Autodesk Inventor part; units mm, degrees
ref_plane "YZ Plane" through (0, 0, 0) normal (1, 0, 0) x (0, 1, 0)
ref_plane "XZ Plane" through (0, 0, 0) normal (0, 1, 0) x (-1, 0, 0)
ref_plane "XY Plane" through (0, 0, 0) normal (0, 0, 1) x (1, 0, 0)
sketch "스케치1" plane through (0, 0, 0) normal (0, 0, 1) x (1, 0, 0)
  line L0 (13.3752, -8.8292) -> (-13.3752, -8.8292)
  line L1 (-13.3752, -8.8292) -> (-13.3752, 8.8292)
  line L2 (-13.3752, 8.8292) -> (13.3752, 8.8292)
  line L3 (13.3752, 8.8292) -> (13.3752, -8.8292)
  line L4 (13.3752, -8.8292) -> (-13.3752, 8.8292) construction
  line L5 (-13.3752, -8.8292) -> (13.3752, 8.8292) construction
  point P0 (0, 0)
extrude "돌출1" add sketch "스케치1" along normal blind 5
sketch "스케치2" plane through (0, 0, 5) normal (0, 0, 1) x (1, 0, 0)
  line L0 (13.3752, 8.8292) -> (-13.3752, 8.8292)
  line L1 (-8.0009, 8.8292) -> (8.3241, 8.8292)
  line L2 (8.3241, 8.8292) -> (8.3241, 5.7582)
  line L3 (8.3241, 5.7582) -> (-8.0009, 5.7582)
  line L4 (-8.0009, 5.7582) -> (-8.0009, 8.8292)
  line L5 (-13.3752, 8.8292) -> (-13.3752, -8.8292)
  line L6 (-13.3752, 1.9598) -> (-7.1927, 1.9598)
  line L7 (-13.3752, -1.5153) -> (-7.1927, -1.5153)
  arc A0 (-7.1927, -1.5153) -> (-7.1927, 1.9598) centre (-6.9174, 0.2222) ccw
  line L8 (13.3752, -8.8292) -> (13.3752, 8.8292)
  line L9 (13.3752, 1.9598) -> (7.2331, 1.9598)
  line L10 (13.3752, -1.5153) -> (7.2331, -1.5153)
  arc A1 (7.2331, 1.9598) -> (7.2331, -1.5153) centre (7.2331, 0.2222) ccw
  point P0 (0, 0)
extrude "돌출2" add sketch "스케치2" along normal blind 10 contours L2 L3 L4 L0
extrude "돌출3" cut sketch "스케치2" against normal blind 10 contours L6 A0 L7 L5 | L8 L10 A1 L9
sketch "스케치3" plane through (-8.0009, 5.7582, 5) normal (0, -1, 0) x (1, 0, 0)
  circle A0 centre (8.0009, 4.1121) radius 2.5125
  line L0 (0, 10) -> (16.325, 10)
  line L1 (0, 0) -> (0, 10)
  arc A1 (8.1625, 10) -> (0, 4.1121) centre (8.0451, 1.5609) ccw
  line L2 (16.325, 0) -> (16.325, 10)
  arc A2 (16.325, 4.1121) -> (8.1625, 10) centre (7.959, 1.1161) ccw
  point P0 (8.0009, -5)
extrude "돌출4" cut sketch "스케치3" against normal blind 10 contours A0
fillet "모깎기1" radius 5 2 edges at (13.3752, -8.8292, 2.5) (-13.3752, -8.8292, 2.5)
sketch "스케치4" plane through (-8.0009, 5.7582, 5) normal (0, -1, 0) x (1, 0, 0)
  point P0 (8.0009, -5)
fillet "모깎기2" radius 7 2 edges at (8.3241, 7.2937, 15) (-8.0009, 7.2937, 15)
properties part number "240531_3Dsketch01"
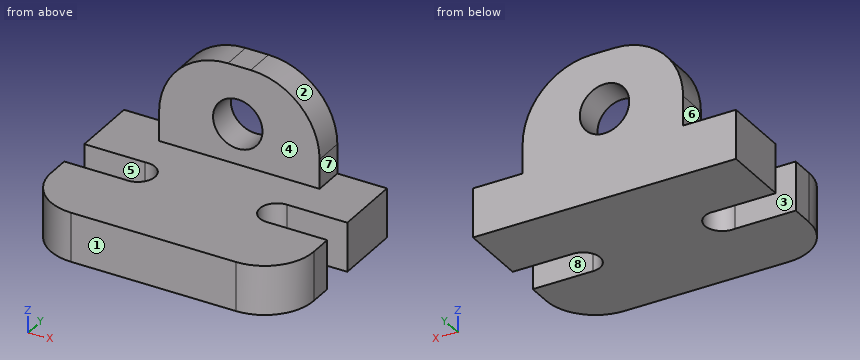
Verification items for the finished model (mm, model axes). Face numbers are marked on the shaded views. A direction names the side the tool comes from. Give positions to 0.01 mm unless a question says otherwise; leave off trailing zeros. Write each loop counter-clockwise with the first axis right and the second up, starting at its lowest first coordinate (ties: lowest second). Pieces come first, ordered by that corner, then holes. Notation, with made-up numbers: (83, 85) - (125, 85) arc R20 ccw to (125, 94) - close; hole circle Ø7 at (47, 34.5). An arc over 180 degrees is marked (long way). Put each result on its own line as item: value.
Q1. Section check C-C on z = 1.25. Record the cut outline in (x, y), and give its area (3 significant figures).
Result:
outline: (-13.38, -3.83) arc R5 ccw to (-8.38, -8.83) - (8.38, -8.83) arc R5 ccw to (13.38, -3.83) - (13.38, -1.52) - (7.23, -1.52) arc R1.74 cw to (7.23, 1.96) - (13.38, 1.96) - (13.38, 8.83) - (-13.38, 8.83) - (-13.38, 1.96) - (-7.19, 1.96) arc R1.76 cw (long way) to (-7.19, -1.52) - (-13.38, -1.52) - close
area: 408 mm2
Q2. Depth check by flat-ended pin: P1, Ø10, axis at x = -6.5, y = -3, coming from the -Z side; P2, Ø1.5, axis at y = 8, z = 7, coming from the +X side; P3, Ø1, axis at x = 5, y = -5, coming from the +Z side; P4, Ø1.5, axis at x = 9.5, z = 3, coming from the -Y side. Enter the tip coordinate at first touch or a pass-through.
Result:
P1: z = 0
P2: x = 8.32
P3: z = 5
P4: y = -8.82
Q3. Mould release check, pull along Y, two halves, no side actions. Record for the marked faces 1, 2 and 3: released by +Y, released by -Y, zero draft, split by the parting line, or undercut.
Result:
face 1: released by -Y
face 2: zero draft
face 3: undercut
Q4. Section check B-B on z = 7. Record the cut outline in (x, y).
Result:
outline: (-8, 5.76) - (-1.36, 5.76) - (-1.36, 8.83) - (-8, 8.83) - close; (1.36, 5.76) - (8.32, 5.76) - (8.32, 8.83) - (1.36, 8.83) - close
Q5. Scan lines: probe 1 along Z at (x, y) = (0, 7.15); probe 2 along Z at (x, y) = (-1.5, 5.5); probe 3 along Y at (x, z) = (-9.75, 1.5). Record each from-to range of solid material in increasing order. Write a range as from..to.
Result:
probe 1: 0..6.6, 11.62..15
probe 2: 0..5
probe 3: -8.64..-1.52, 1.96..8.83
Q6. Set-up check for the marked faces 4, 5, 6, 7 and 8: record each of +Z, -Z, +X, -X, +Y, -Y from which the full face is reachable in a straight line by a thin tool's end or side.
Result:
face 4: +Z, +X, -X, -Y
face 5: +Z, -Z, -X
face 6: +Z, -X, +Y, -Y
face 7: +Z, +X, +Y, -Y
face 8: +Z, -Z, +X
Q7. Section check A-A on x = 0. Record the cut outline in (y, z).
Result:
outline: (-8.83, 0) - (8.83, 0) - (8.83, 6.6) - (5.76, 6.6) - (5.76, 5) - (-8.83, 5) - close; (5.76, 11.62) - (8.83, 11.62) - (8.83, 15) - (5.76, 15) - close
Q8. Section check D-D on y = 3.75. Record the cut outline in (x, z), and give its area (3 significant figures).
Result:
outline: (-13.38, 0) - (13.38, 0) - (13.38, 5) - (-13.38, 5) - close
area: 134 mm2
